Here's the drawing with two shaded views (mm, measured from the low corner). I have some questions. A direction names the side the tool comes from. Give positions to 0.01 mm unless a question says otherwise; leave off trailing zeros. Loops run counter-clockwise (first coordinate to the right, second up) from the corner with the lowest first, then second, coordinate; pieces in that order, holes last.
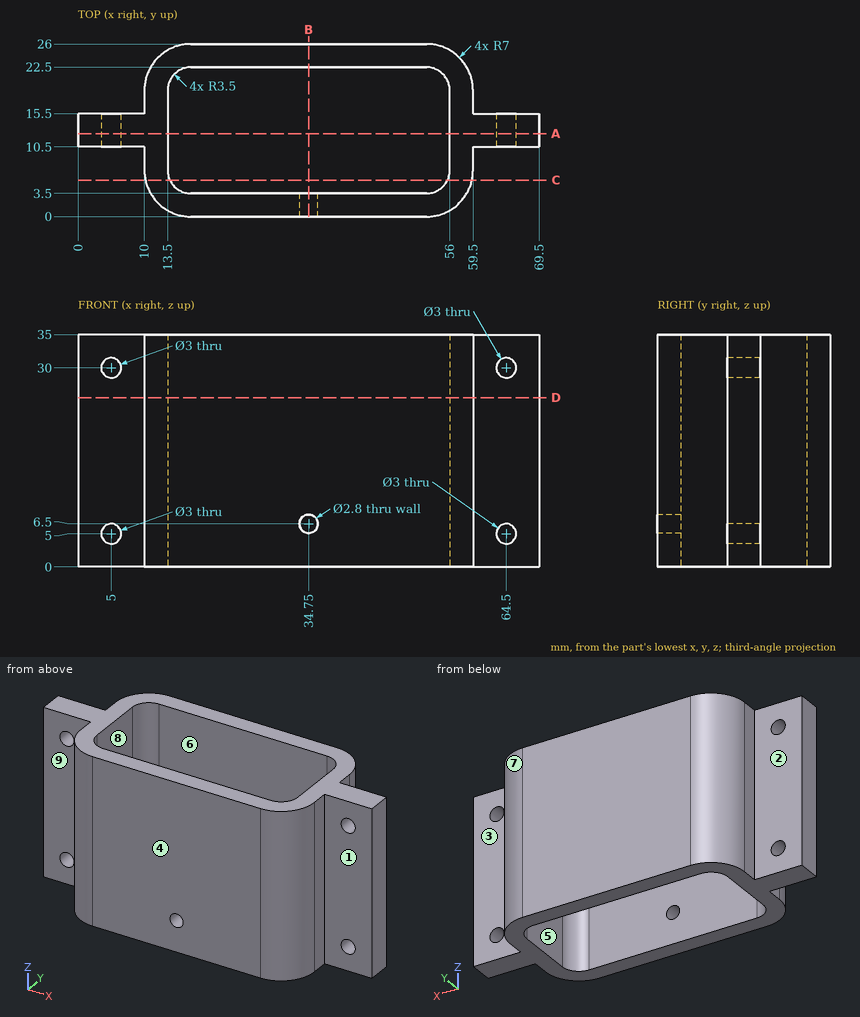
(1) Thinking about a two-plate mould opening in X: for the marked faces 6, 7, 8 and 9, which applies, pulls with the +X half, pulls with the -X half, needs draft (parallel to the pull), parting line crosses it, or undercut?
Returned:
face 6: undercut
face 7: pulls with the +X half
face 8: undercut
face 9: needs draft
(2) Suppose I cut it at B-B on x = 34.75. List the corners of the cut face in (y, z) for me, plus the area to 3 significant figures.
Returned:
outline: (0, 0) - (3.5, 0) - (3.5, 5.1) - (0, 5.1) - close; (0, 7.9) - (3.5, 7.9) - (3.5, 35) - (0, 35) - close; (22.5, 0) - (26, 0) - (26, 35) - (22.5, 35) - close
area: 235 mm2
(3) Which directions (+Z, -Z, +X, -X, +Y, -Y) give clear straight access to the entire face, cutting with the end or side of a thin tool? Please do the marked faces 1, 2, 3, 4 and 5.
Returned:
face 1: +Z, -Z, +X, -Y
face 2: +Z, -Z, -X, +Y
face 3: +Z, -Z, +X, +Y
face 4: +Z, -Z, +X, -X, -Y
face 5: +Z, -Z
(4) Please list where these lines run through material, in increasing order: probe 1 along Z at (x, y) = (5, 12.7); probe 2 along Y at (x, z) = (38, 11); probe 3 along Z at (x, y) = (34.75, 2.25).
Returned:
probe 1: z = 0 to 3.5, 6.5 to 28.5, 31.5 to 35
probe 2: y = 0 to 3.5, 22.5 to 26
probe 3: z = 0 to 5.1, 7.9 to 35
(5) Will these pins go through, and if not, where does the flat tip stop? P1, Ø9.5, axis at y = 15, z = 15, coming from the -X side; P2, Ø5, axis at x = 2.5, z = 16, coming from the -Y side; P3, Ø11, axis at x = 63.5, z = 16.5, coming from the +Y side; P4, Ø5, axis at y = 18.5, z = 15, coming from the -X side.
Returned:
P1: stops at x = 0
P2: stops at y = 10.5
P3: stops at y = 23.33
P4: stops at x = 10
(6) Suppose I cut it at D-D on z = 25.5. List the corners of the cut face in (x, y) for me, plus the area to 3 significant figures.
Returned:
outline: (0, 10.5) - (10, 10.5) - (10, 7) arc R7 ccw to (17, 0) - (52.5, 0) arc R7 ccw to (59.5, 7) - (59.5, 10.5) - (69.5, 10.5) - (69.5, 15.5) - (59.5, 15.5) - (59.5, 19) arc R7 ccw to (52.5, 26) - (17, 26) arc R7 ccw to (10, 19) - (10, 15.5) - (0, 15.5) - close; hole (13.5, 7) arc R3.5 ccw to (17, 3.5) - (52.5, 3.5) arc R3.5 ccw to (56, 7) - (56, 19) arc R3.5 ccw to (52.5, 22.5) - (17, 22.5) arc R3.5 ccw to (13.5, 19) - close
area: 548 mm2
(7) Suppose I cut it at A-A on y = 12.5. List the corners of the cut face in (x, z) for me, plus the area to 3 significant figures.
Returned:
outline: (0, 0) - (13.5, 0) - (13.5, 35) - (0, 35) - close; (56, 0) - (69.5, 0) - (69.5, 35) - (56, 35) - close; hole circle Ø3 at (5, 5); hole circle Ø3 at (5, 30); hole circle Ø3 at (64.5, 5); hole circle Ø3 at (64.5, 30)
area: 917 mm2
(8) Suppose I cut it at C-C on y = 5.5. List the corners of the cut face in (x, z) for me.
Returned:
outline: (10.16, 0) - (13.84, 0) - (13.84, 35) - (10.16, 35) - close; (55.66, 0) - (59.34, 0) - (59.34, 35) - (55.66, 35) - close
